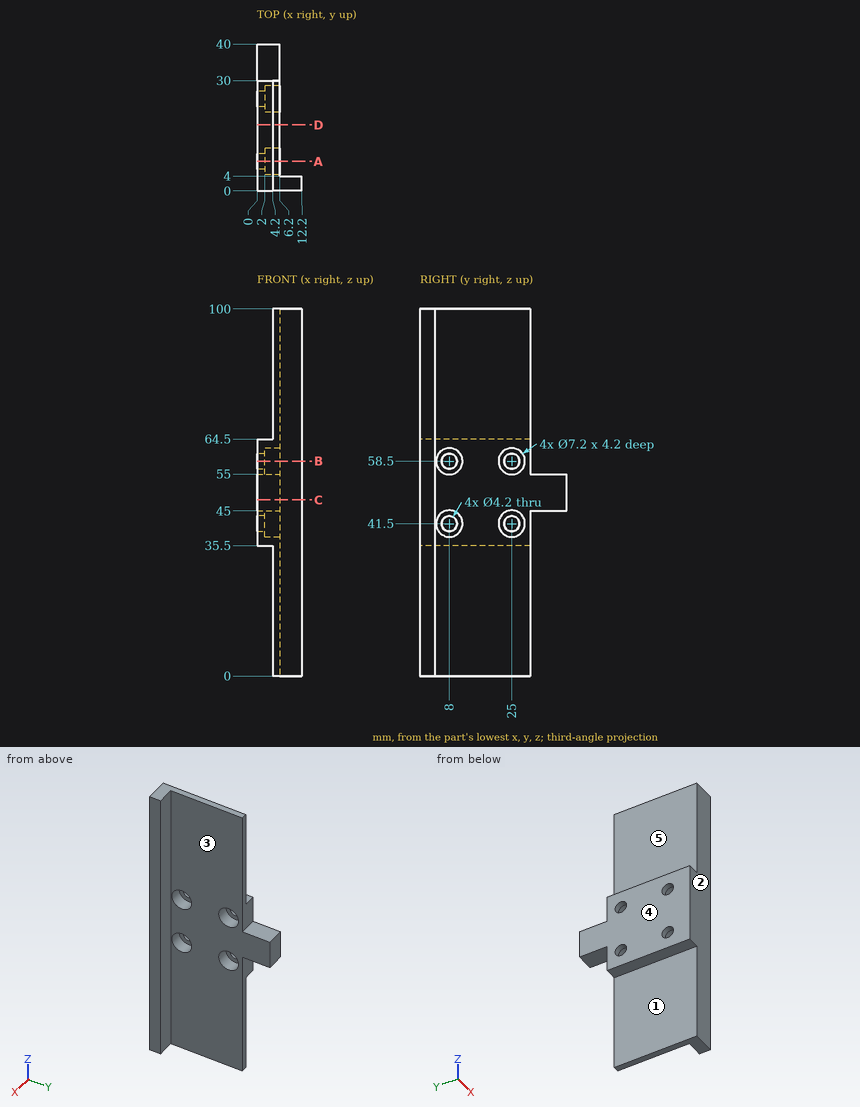
Answer from the drawing. Dimensions are ordinates in mm from the lowest x, y and z of the part. A direction names the side the tool comes from. Give positions to 0.01 mm unless a question says otherwise; leave off trailing zeros. Loops run counter-clockwise (first coordinate to the right, second up) from the corner with the lowest first, then second, coordinate; pieces in that order, holes last. Notation, with made-up numbers: (53.25, 14) - (103.25, 14) arc R26 cw to (103.25, 33) - close; hole circle Ø1 at (51, 82). An arc over 180 degrees is marked (long way). Write each question's results on one line, items separated by ' | '.
1. Find section C-C, the plane z = 48. Write down the section's boundary in (x, y), then the cut area to 3 significant figures.
Resolved:
outline: (0, 0) - (12.2, 0) - (12.2, 4) - (6.2, 4) - (6.2, 40) - (0, 40) - close | area: 272 mm^2
2. Which of the six approach directions +Z, -Z, +X, -X, +Y, -Y give full straight-line access (tool end or side, diameter ignored) to the marked faces 1, 2, 3, 4 and 5?
Resolved:
face 1: -Z, -X, +Y, -Y | face 2: +Z, -Z, +X, -X, -Y | face 3: +Z, -Z, +X, +Y | face 4: +Z, -Z, -X, +Y, -Y | face 5: +Z, -X, +Y, -Y
3. Find section A-A, the plane y = 8. Write down the section's boundary in (x, z), then the cut area to 3 significant figures.
Resolved:
outline: (0, 35.5) - (4.2, 35.5) - (4.2, 0) - (6.2, 0) - (6.2, 37.9) - (2, 37.9) - (2, 39.4) - (0, 39.4) - close; (0, 43.6) - (2, 43.6) - (2, 45.1) - (6.2, 45.1) - (6.2, 54.9) - (2, 54.9) - (2, 56.4) - (0, 56.4) - close; (0, 60.6) - (2, 60.6) - (2, 62.1) - (6.2, 62.1) - (6.2, 100) - (4.2, 100) - (4.2, 64.5) - (0, 64.5) - close | area: 245 mm^2
4. Flat-ended cylindrical pins translate along their axes: P1, Ø1.9, axis at x = 2.5, y = 33.5, coming from the +Z side; P2, Ø6.5, axis at y = 8, z = 58.5, coming from the +X side; P3, Ø1.9, axis at x = 3, y = 37, coming from the -Z side; P4, Ø2, axis at y = 25, z = 58, coming from the +X side. Find the tip coordinate at first contact, or state that the pin passes through.
Resolved:
P1: stops at z = 55 | P2: stops at x = 2 | P3: stops at z = 45 | P4: passes through
5. Find section D-D, the plane y = 18. Write down the section's boundary in (x, z), then the cut area to 3 significant figures.
Resolved:
outline: (0, 35.5) - (4.2, 35.5) - (4.2, 0) - (6.2, 0) - (6.2, 100) - (4.2, 100) - (4.2, 64.5) - (0, 64.5) - close | area: 322 mm^2
6. Consider probe 1 along Y at (x, z) = (4.6, 41.5); probe 2 along Y at (x, z) = (1.15, 41.5); probe 3 along Z at (x, y) = (4.5, 22). Determine where each line is inside the solid, lowest interval first. Write a range as from..to.
Resolved:
probe 1: y = 0..4.4, 11.6..21.4, 28.6..30 | probe 2: y = 0..5.9, 10.1..22.9, 27.1..30 | probe 3: z = 0..39.51, 43.49..56.51, 60.49..100
7. Find section B-B, the plane z = 58.5. Write down the section's boundary in (x, y).
Resolved:
outline: (0, 0) - (12.2, 0) - (12.2, 4) - (6.2, 4) - (6.2, 4.4) - (2, 4.4) - (2, 5.9) - (0, 5.9) - close; (0, 10.1) - (2, 10.1) - (2, 11.6) - (6.2, 11.6) - (6.2, 21.4) - (2, 21.4) - (2, 22.9) - (0, 22.9) - close; (0, 27.1) - (2, 27.1) - (2, 28.6) - (6.2, 28.6) - (6.2, 30) - (0, 30) - close
